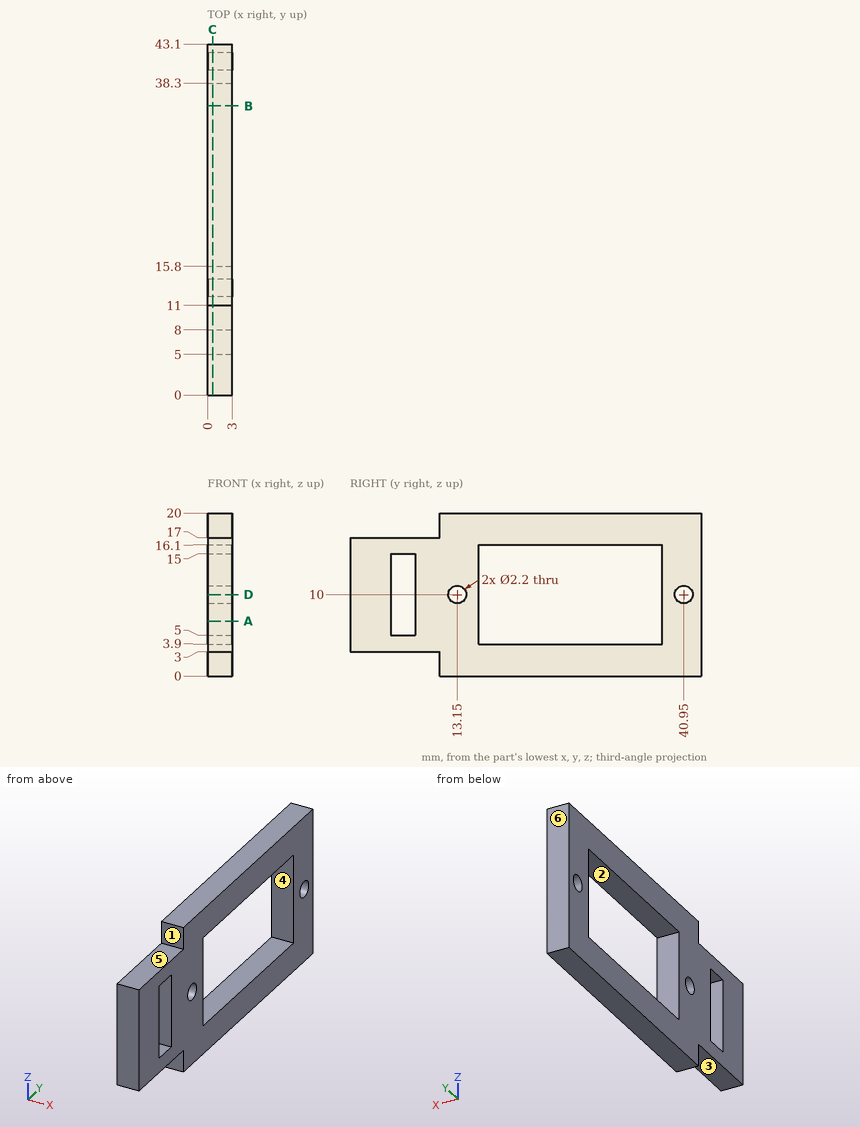
For this review, use the dimensioned drawing (mm, ordinates from the lowest corner) and the shaded views. A direction names the side the tool comes from. Coordinates: 2 decimals unless noted, no trailing zeros. Loops run counter-clockwise (first coordinate to the right, second up) from the corner with the lowest first, then second, coordinate; pieces in that order, holes last. Notation, with made-up numbers: (-24.75, 7.25) - (32.25, 7.25) arc R21 ccw to (32.25, 35.25) - close; hole circle Ø1 at (58.5, -0.5). An arc over 180 degrees is marked (long way). Use CSV: the item, a comma, the result in double quotes. Start each with the question number.
1) Tool access review of the marked faces 1, 2 and 3: name each direction out of +Z, -Z, +X, -X, +Y, -Y from which nothing blocks a thin tool from reaching the whole face with its end or side.
2) For pin 1 Ø1.5 at (x, z) = (1.5, 18) entering from -Y; pin 2 Ø1.5 at (x, y) = (1.5, 3.5) entering from +Z; pin 3 Ø0.9 at (x, y) = (1, 4) entering from -Z; pin 4 Ø1.3 at (y, z) = (40.95, 10) entering from +X, all flat-tipped, find the tip position at first contact; note any pin that passes through.
3) Consider section C-C on x = 0.6. Write out the cut boundary in (y, z).
4) Consider section B-B on y = 35.5. Write out the cut boundary in (x, z), then the cut area to 3 significant figures.
5) Consider section D-D on z = 10. Write out the cut boundary in (x, y), then the cut area to 3 significant figures.
6) The part is to be moulded in two halves that separate along Z. For the marked faces 4, 5 and 6, say which applies: +Z half, -Z half, draft (parallel to the pull), parting line (faces both ways), or undercut.
7) Wall thickness on L1, parallel to Y at x = 2, z = 10; L2, parallel to Y at x = 0.4, z = 7.75; L3, parallel to Z at x = 0.75, y = 18: over which ranges is each line inside the solid? List them lowest first. Write a range as from..to.
8) Consider section A-A on z = 6.75. Write out the cut boundary in (x, y).
Geometry says:
1,face 1,"+Z, +X, -X, -Y"
1,face 2,"+X, -X"
1,face 3,"-Z, +X, -X, -Y"
2,pin 1,"y = 11"
2,pin 2,"z = 17"
2,pin 3,"z = 3"
2,pin 4,"through"
3,outline,"(0, 3) - (11, 3) - (11, 0) - (43.1, 0) - (43.1, 20) - (11, 20) - (11, 17) - (0, 17) - close; hole (5, 5) - (8, 5) - (8, 15) - (5, 15) - close; hole circle Ø2.2 at (13.15, 10); hole (15.8, 3.9) - (38.3, 3.9) - (38.3, 16.1) - (15.8, 16.1) - close; hole circle Ø2.2 at (40.95, 10)"
4,outline,"(0, 0) - (3, 0) - (3, 3.9) - (0, 3.9) - close; (0, 16.1) - (3, 16.1) - (3, 20) - (0, 20) - close"
4,area,"23.4 mm^2"
5,outline,"(0, 0) - (3, 0) - (3, 5) - (0, 5) - close; (0, 8) - (3, 8) - (3, 12.05) - (0, 12.05) - close; (0, 14.25) - (3, 14.25) - (3, 15.8) - (0, 15.8) - close; (0, 38.3) - (3, 38.3) - (3, 39.85) - (0, 39.85) - close; (0, 42.05) - (3, 42.05) - (3, 43.1) - (0, 43.1) - close"
5,area,"39.6 mm^2"
6,face 4,"undercut"
6,face 5,"+Z half"
6,face 6,"draft"
7,L1,"0..5, 8..12.05, 14.25..15.8, 38.3..39.85, 42.05..43.1"
7,L2,"0..5, 8..15.8, 38.3..43.1"
7,L3,"0..3.9, 16.1..20"
8,outline,"(0, 0) - (3, 0) - (3, 5) - (0, 5) - close; (0, 8) - (3, 8) - (3, 15.8) - (0, 15.8) - close; (0, 38.3) - (3, 38.3) - (3, 43.1) - (0, 43.1) - close"
